The model under review builds one solid part; all positions refer to its coordinate system, in mm. A direction names the side the tool comes from. Give positions to 0.01 mm unless a question says otherwise; leave off trailing zeros. Loops run counter-clockwise (first coordinate to the right, second up) from the corner with the lowest first, then second, coordinate; pieces in that order, holes last. Notation, with made-up numbers: M 88,-17.75 L 94,-17.75 A21 ccw 94,8.25 Z; hole C 8,-29.75 d5. An arc over 180 degrees is marked long. Write item = value, one per line. Start each with the question number.
1. For faces 1 (the face through (0, -21, 30)), 2 (the face through (12.5, 0.07, 98.03)), 3 (the face through (0, 3, 111)), list the 3-axis set-ups (+Z, -Z, +X, -X, +Y, -Y) from which the entire face can be reached by the end or side of a thin tool; tool diameter is ignored.
2. For pin 1 (2.5 mm diameter, centred on x = 0, y = 14, fed in from +Z); pin 2 (4 mm diameter, centred on x = -0.5, z = 109.5, fed in from +Y); pin 3 (3.5 mm diameter, centred on x = 0.5, y = 14.5, fed in from +Z), all flat-tipped, find the tip position at first contact; note any pin that passes through.
3. We need section C-C on x = -6. Give the boundary of the cut face in (y, z).
4. We need section B-B on x = 0. Give the boundary of the cut face in (y, z), then the cut area to 3 significant figures.
5. We need section A-A on y = 0. Give the boundary of the cut face in (x, z).
6. We need section D-D on y = -6.5. Give the boundary of the cut face in (x, z).
7. Wall thickness on line 1 along Y through (x, z) = (0, 98); line 2 along Y through (x, z) = (14, 98); line 3 along Z through (x, y) = (11.5, -10): over which ranges is each line inside the solid? List them lowest first. Write a range as from..to.
8. Draft analysis for pull direction X (two halves, no side actions). For faces 4 (the face through (-8, -8, 100)), 5 (the face through (-0.325, 12.536, 98.028)), 6 (the face through (-2.38, -10.74, 100.99)), 7 (the face through (0, 14, 96)), state which applies: pulls with the +X half, pulls with the -X half, needs draft (parallel to the pull), parting line crosses it, or undercut.
from build123d import *

# Parameters (mm, degrees)
SKETCH_1_W          = 42
SKETCH_1_H          = 42
EXTRUDE_1_DEPTH     = 60
SKETCH_2_R          = 18
EXTRUDE_2_DEPTH     = 40
SKETCH_3_R          = 11
EXTRUDE_3_DEPTH     = 2
SKETCH_4_R          = 4
EXTRUDE_4_DEPTH     = 17
SKETCH_5_R          = 1.5
CUT_EXTRUDE_1_DEPTH = 4
CUT_EXTRUDE_START   = -15
CUT_EXTRUDE_2_DEPTH = 15


with BuildPart() as part:
    # 草图1 → 凸台-拉伸1 (new body)
    with BuildSketch(Plane.XY):
        Rectangle(SKETCH_1_W, SKETCH_1_H)
    extrude(amount=EXTRUDE_1_DEPTH)

    # 草图2 → 凸台-拉伸2 (add)
    with BuildSketch(Plane.XY.offset(60)):
        Circle(SKETCH_2_R)
    extrude(amount=EXTRUDE_2_DEPTH)

    # 草图3 → 凸台-拉伸3 (add)
    with BuildSketch(Plane.XY.offset(100)):
        Circle(SKETCH_3_R)
    extrude(amount=EXTRUDE_3_DEPTH)

    # 草图4 → 凸台-拉伸4 (add)
    with BuildSketch(Plane.XY.offset(102)):
        Circle(SKETCH_4_R)
    extrude(amount=EXTRUDE_4_DEPTH)

    # 草图5 → 切除-拉伸1 (cut)
    with BuildSketch(Plane.XY.offset(100)):
        with Locations((0, 14)):
            Circle(SKETCH_5_R)
        with Locations((14, 0)):
            Circle(SKETCH_5_R)
        with Locations((0, -14)):
            Circle(SKETCH_5_R)
        with Locations((-14, 0)):
            Circle(SKETCH_5_R)
    extrude(amount=-CUT_EXTRUDE_1_DEPTH, mode=Mode.SUBTRACT)

    # 草图6 → 切除-拉伸2 (cut)
    with BuildSketch(Plane.XY.offset(119).offset(CUT_EXTRUDE_START)):
        with BuildLine():
            Line((2.645751311, 3), (-2.645751311, 3))
            ThreePointArc((-2.645751311, 3), (0, 4), (2.645751311, 3))
        make_face()
    extrude(amount=CUT_EXTRUDE_2_DEPTH, mode=Mode.SUBTRACT)


solid = part.part
Final values:
q1.face_1 = +Z, -Z, +X, -X, -Y
q1.face_2 = +Z
q1.face_3 = +Z, +X, -X, +Y
q2.pin_1 = 96
q2.pin_2 = 3
q2.pin_3 = 100
q3.outline = M -21,0 L 21,0 L 21,60 L 16.97,60 L 16.97,100 L 9.22,100 L 9.22,102 L -9.22,102 L -9.22,100 L -16.97,100 L -16.97,60 L -21,60 Z
q4.outline = M -21,0 L 21,0 L 21,60 L 18,60 L 18,100 L 15.5,100 L 15.5,96 L 12.5,96 L 12.5,100 L 11,100 L 11,102 L 4,102 L 4,104 L 3,104 L 3,119 L -4,119 L -4,102 L -11,102 L -11,100 L -12.5,100 L -12.5,96 L -15.5,96 L -15.5,100 L -18,100 L -18,60 L -21,60 Z
q4.area = 4,100 mm²
q5.outline = M -21,0 L 21,0 L 21,60 L 18,60 L 18,100 L 15.5,100 L 15.5,96 L 12.5,96 L 12.5,100 L 11,100 L 11,102 L 4,102 L 4,119 L -4,119 L -4,102 L -11,102 L -11,100 L -12.5,100 L -12.5,96 L -15.5,96 L -15.5,100 L -18,100 L -18,60 L -21,60 Z
q6.outline = M -21,0 L 21,0 L 21,60 L 16.79,60 L 16.79,100 L 8.87,100 L 8.87,102 L -8.87,102 L -8.87,100 L -16.79,100 L -16.79,60 L -21,60 Z
q7.line_1 = -18..-15.5, -12.5..12.5, 15.5..18
q7.line_2 = -11.31..-1.5, 1.5..11.31
q7.line_3 = 0..100
q8.face_4 = needs draft
q8.face_5 = undercut
q8.face_6 = parting line crosses it
q8.face_7 = undercut
